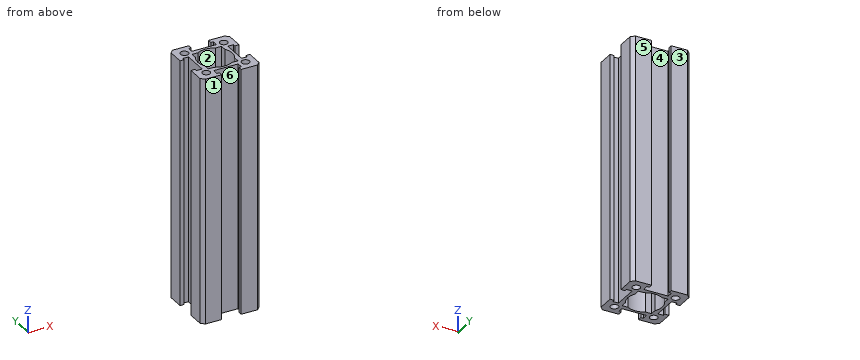
from build123d import *

# Parameters (mm, degrees)
SKETCH1_R           = 1.6
BOSS_EXTRUDE1_DEPTH = 100


with BuildPart() as part:
    # Sketch1 → Boss-Extrude1 (new body)
    with BuildSketch(Plane.XY):
        with BuildLine():
            Line((-8, -5), (-10.291177135, -5))
            Line((-10.291177135, -5), (-10.291177135, -4))
            Line((-10.291177135, -4), (-12, -4))
            Line((-12, -4), (-12, -10.583005244))
            ThreePointArc((-12, -10.583005244), (-11.313708499, -11.313708499), (-10.583005244, -12))
            Line((-10.583005244, -12), (-4, -12))
            Line((-4, -12), (-4, -10.291177135))
            Line((-4, -10.291177135), (-5, -10.291177135))
            Line((-5, -10.291177135), (-5, -8))
            Line((-5, -8), (5, -8))
            Line((5, -8), (5, -10.291177135))
            Line((5, -10.291177135), (4, -10.291177135))
            Line((4, -10.291177135), (4, -12))
            Line((4, -12), (10.583005244, -12))
            ThreePointArc((10.583005244, -12), (11.313708499, -11.313708499), (12, -10.583005244))
            Line((12, -10.583005244), (12, -4))
            Line((12, -4), (10.291177135, -4))
            Line((10.291177135, -4), (10.291177135, -5))
            Line((10.291177135, -5), (8, -5))
            Line((8, -5), (8, 5))
            Line((8, 5), (10.291177135, 5))
            Line((10.291177135, 5), (10.291177135, 4))
            Line((10.291177135, 4), (12, 4))
            Line((12, 4), (12, 10.583005244))
            ThreePointArc((12, 10.583005244), (11.313708499, 11.313708499), (10.583005244, 12))
            Line((10.583005244, 12), (4, 12))
            Line((4, 12), (4, 10.291177135))
            Line((4, 10.291177135), (5, 10.291177135))
            Line((5, 10.291177135), (5, 8))
            Line((5, 8), (-5, 8))
            Line((-5, 8), (-5, 10.291177135))
            Line((-5, 10.291177135), (-4, 10.291177135))
            Line((-4, 10.291177135), (-4, 12))
            Line((-4, 12), (-10.583005244, 12))
            ThreePointArc((-10.583005244, 12), (-11.313708499, 11.313708499), (-12, 10.583005244))
            Line((-12, 10.583005244), (-12, 4))
            Line((-12, 4), (-10.291177135, 4))
            Line((-10.291177135, 4), (-10.291177135, 5))
            Line((-10.291177135, 5), (-8, 5))
            Line((-8, 5), (-8, -5))
        make_face()
        with Locations((-8, -8)):
            Circle(SKETCH1_R, mode=Mode.SUBTRACT)
        with Locations((8, 8)):
            Circle(SKETCH1_R, mode=Mode.SUBTRACT)
        with Locations((-8, 8)):
            Circle(SKETCH1_R, mode=Mode.SUBTRACT)
        with Locations((8, -8)):
            Circle(SKETCH1_R, mode=Mode.SUBTRACT)
        with BuildLine():
            Line((-3.605551275, -6), (-6, -6))
            Line((-6, -6), (-6, -3.605551275))
            ThreePointArc((-6, -3.605551275), (-7, 0), (-6, 3.605551275))
            Line((-6, 3.605551275), (-6, 6))
            Line((-6, 6), (-3.605551275, 6))
            ThreePointArc((-3.605551275, 6), (0, 7), (3.605551275, 6))
            Line((3.605551275, 6), (6, 6))
            Line((6, 6), (6, 3.605551275))
            ThreePointArc((6, 3.605551275), (7, 0), (6, -3.605551275))
            Line((6, -3.605551275), (6, -6))
            Line((6, -6), (3.605551275, -6))
            ThreePointArc((3.605551275, -6), (0, -7), (-3.605551275, -6))
        make_face(mode=Mode.SUBTRACT)
    extrude(amount=BOSS_EXTRUDE1_DEPTH)


solid = part.part
Read the model definition and answer for the solid it produces. Units are mm, in the model's axes. Face numbers are marked on the shaded views. A direction names the side the tool comes from. Round coordinates to 2 decimals unless told otherwise and drop trailing zeros. Loops run counter-clockwise (first coordinate to the right, second up) from the corner with the lowest first, then second, coordinate; pieces in that order, holes last. Notation, with made-up numbers: (26, -20) - (55, -20) arc R24 ccw to (55, -6) - close; hole circle Ø9 at (32.5, 32.5). An arc over 180 degrees is marked (long way). One line per question, with ' | ' between items. Start each with the question number.
Q1. Find the intervals of material crossed by L1, parallel to X at y = -8.25, z = 77; L2, parallel to X at y = -10.5, z = 54; L3, parallel to X at y = 0.5, z = 62, in increasing order.
Q2. Section A-A on y = -2.75 is taken. Give the vertices of the cut face in (x, z), plus the area to 3 significant figures.
Q3. For a pull along Y with two mould halves and no side action, classify the marked faces 1, 2, 3 and 4 as +Y half, -Y half, draft (parallel to the pull), parting line (faces both ways), or undercut.
Q4. Section B-B on z = 75 is taken. Count the separate pieces of the cut face and the enclosed holes in it, plus the area to 3 significant figures.
Q5. For the marked faces 5 and 6, determine the directions among +Z, -Z, +X, -X, +Y, -Y from which every point of the face is accessible in a straight line to the end or side of a thin tool.
Q6. Flat-ended cylindrical pins translate along their axes: pin 1 (4 mm diameter, centred on x = 1.5, z = 52.5, fed in from -Y); pin 2 (0.5 mm diameter, centred on y = -11, z = 49, fed in from +X); pin 3 (0.5 mm diameter, centred on y = -11, z = 69.5, fed in from -X). Find the tip coordinate at first contact, or state that the pin passes through.
Established:
1) L1: -12 to -9.58, -6.42 to -5, 5 to 6.42, 9.58 to 12 | L2: -12 to -4, 4 to 12 | L3: -8 to -6.98, 6.98 to 8
2) outline: (-8, 0) - (-6.44, 0) - (-6.44, 100) - (-8, 100) - close; (6.44, 0) - (8, 0) - (8, 100) - (6.44, 100) - close | area: 313 mm²
3) face 1: -Y half | face 2: undercut | face 3: +Y half | face 4: undercut
4) separate pieces: 1 | enclosed holes: 5 | area: 230 mm²
5) face 5: +Z, -Z, +X, -X, +Y | face 6: +Z, -Z
6) pin 1: y = -8 | pin 2: x = 11.85 | pin 3: x = -11.85
